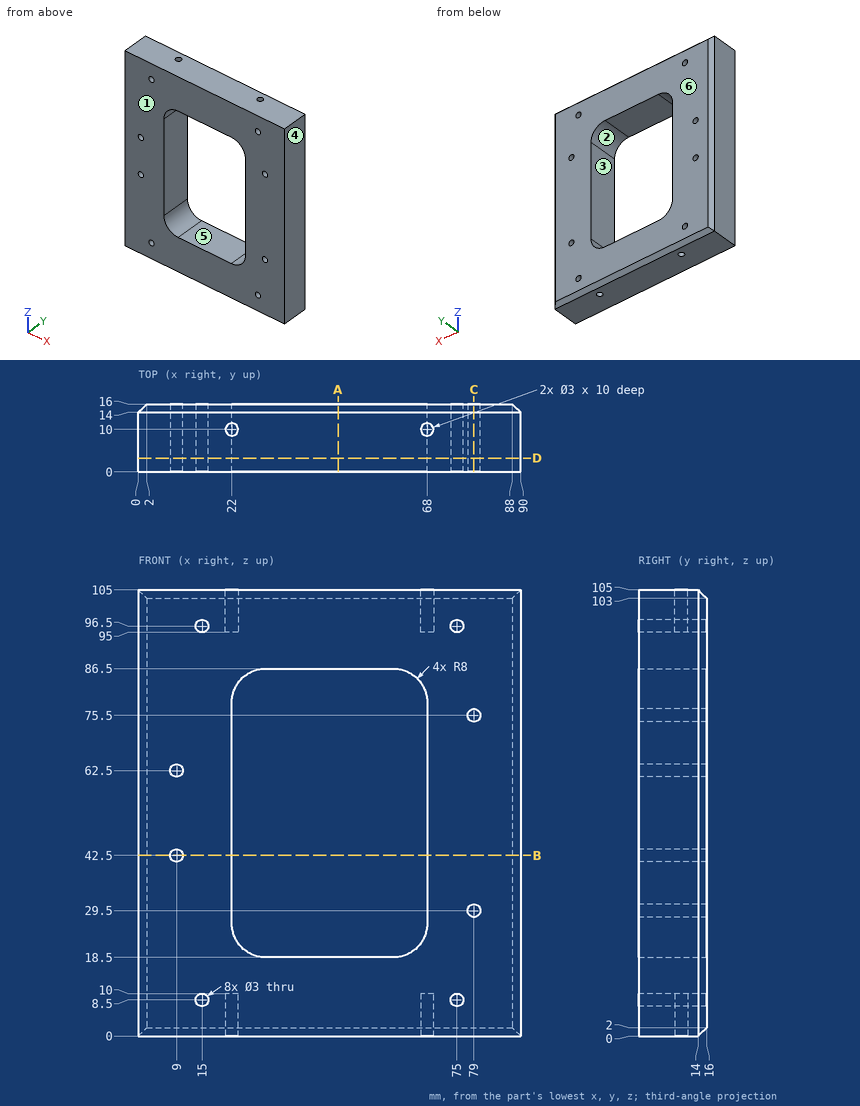
For this review, use the dimensioned drawing (mm, ordinates from the lowest corner) and the shaded views. A direction names the side the tool comes from. Give positions to 0.01 mm unless a question says otherwise; leave off trailing zeros. Order: outer loops, then holes, each group sorted by start corner. A loop starts at its lowest first (then second) coordinate and runs counter-clockwise, first axis right, second up. Notation, with made-up numbers: (-17.75, 10.25) -> (37.25, 10.25) arc R11 cw to (37.25, 16.25) -> close; hole circle Ø7 at (-28.75, 29.5). An arc over 180 degrees is marked (long way). Write item = value, one per line. Start each with the question number.
(1) Take a section at C-C (x = 79). Write out the cut boundary in (y, z).
(2) For L1, parallel to X at y = 5.25, z = 29.5; L2, parallel to X at y = 12.75, z = 8.5; L3, parallel to Z at x = 9, y = 11.5, list the stretches that pass through material, from the lowest coordinate up. Write a range as from..to.
(3) Tool access review of the marked faces 5 and 6: name each direction out of +Z, -Z, +X, -X, +Y, -Y from which nothing blocks a thin tool from reaching the whole face with its end or side.
(4) Take a section at D-D (y = 3.25). State how many separate pieces and enclosed holes the cut face has, plus the area to 3 significant figures.
(5) Take a section at A-A (x = 47). Write out the cut boundary in (y, z).
(6) Take a section at B-B (z = 42.5). Write out the cut boundary in (x, y), plus the area to 3 significant figures.
(7) Draft analysis for pull direction X (two halves, no side actions). For the marked faces 1, 2, 3 and 4, state which applies: +X half, -X half, draft (parallel to the pull), parting line (faces both ways), or undercut.
(8) For pin 1 Ø2.5 at (x, y) = (22, 10) entering from -Z; pin 2 Ø2.5 at (x, z) = (15, 8.5) entering from +Y; pin 3 Ø0.9 at (x, y) = (67.5, 10) entering from +Z, all flat-tipped, find the tip position at first contact; note any pin that passes through.
Returned:
q1.outline = (0, 0) -> (14, 0) -> (16, 2) -> (16, 28) -> (0, 28) -> close; (0, 31) -> (16, 31) -> (16, 74) -> (0, 74) -> close; (0, 77) -> (16, 77) -> (16, 103) -> (14, 105) -> (0, 105) -> close
q2.L1 = 0..22, 68..77.5, 80.5..90
q2.L2 = 0..13.5, 16.5..73.5, 76.5..90
q2.L3 = 0..41, 44..61, 64..105
q3.face_5 = +Y, -Y
q3.face_6 = +Z, -Z, +X, -X, +Y
q4.separate_pieces = 1
q4.enclosed_holes = 9
q4.area = 6,320 mm²
q5.outline = (0, 0) -> (14, 0) -> (16, 2) -> (16, 18.5) -> (0, 18.5) -> close; (0, 86.5) -> (16, 86.5) -> (16, 103) -> (14, 105) -> (0, 105) -> close
q6.outline = (0, 0) -> (7.5, 0) -> (7.5, 16) -> (2, 16) -> (0, 14) -> close; (10.5, 0) -> (22, 0) -> (22, 16) -> (10.5, 16) -> close; (68, 0) -> (90, 0) -> (90, 14) -> (88, 16) -> (68, 16) -> close
q6.area = 652 mm²
q7.face_1 = draft
q7.face_2 = undercut
q7.face_3 = undercut
q7.face_4 = +X half
q8.pin_1 = 10
q8.pin_2 = through
q8.pin_3 = 95
